from build123d import *

# Parameters (mm, degrees)
F0_R     = 6.35
F1_DEPTH = 12.7
F2_R     = 3.175
F3_DEPTH = 25.4
F4_SIZE  = 3.17499
F5_R     = 3.175
F6_DEPTH = 12.7


# Not quite as in the source:
# - a fillet or chamfer is up to 0.001 mm smaller than in the source, because OpenCascade refuses the exact size


with BuildPart() as f1:
    # F0 (on Top) → F1 (new body, symmetric)
    with BuildSketch(Plane.XY):
        Circle(F0_R)
    extrude(amount=F1_DEPTH, both=True)

    # F2 (on Top) → F3 (join, symmetric)
    with BuildSketch(Plane.XY):
        Circle(F2_R)
    extrude(amount=F3_DEPTH, both=True)

    # F4 (size 3.175 in the source; OpenCascade refuses exactly that, so slightly less here)
    f4_edges = [f1.edges().sort_by_distance(p)[0] for p in [
        (-6.35, 0, -12.7),
        (-6.35, 0, 12.7),
    ]]
    chamfer(f4_edges, length=F4_SIZE)

    # F5 (on Right) → F6 (cut, symmetric)
    with BuildSketch(Plane.YZ):
        Circle(F5_R)
    extrude(amount=F6_DEPTH, both=True, mode=Mode.SUBTRACT)


solid = f1.part
Check sheet for the modelled part. Datum: model origin and axes. Units: mm. A direction names the side the tool comes from. Coordinates: 2 decimals unless noted, no trailing zeros. Loops run counter-clockwise (first coordinate to the right, second up) from the corner with the lowest first, then second, coordinate; pieces in that order, holes last. Notation, with made-up numbers: (-0.75, 19) -> (40.25, 19) arc R34 ccw to (40.25, 57) -> close; hole circle Ø8 at (-18, 17.5). An arc over 180 degrees is marked (long way). Write item = value, one per line. Start each with the question number.
1. Section check C-C on z = 19. Record the cut outline in (x, y) (3 decimals), then the cut area to 3 significant figures.
2. Section check D-D on z = 0. Record the cut outline in (x, y) (3 decimals).
3. Material ranges on line 1 (Z direction, x = -2.75, y = 0) (3 decimals); line 2 (Z direction, x = 1.25, y = 2.5); line 3 (Y direction, x = -1.5, z = 0) (3 decimals), recorded low to high.
4. Depth check by flat-ended pin: P1, Ø5, axis at x = 3, y = -5, coming from the -Z side; P2, Ø3, axis at x = -5, z = 9.5, coming from the +Y side; P3, Ø2, axis at x = 2.5, y = 4.5, coming from the -Z side; P4, Ø5.5, axis at y = 0, z = 0, coming from the +X side. Enter the tip coordinate at first touch or a pass-through.
5. Tool access check on faces 4 (the cylindrical face through (-5.04, -3.86, 0.13)), 5 (the cylindrical face through (-0.69, -3.1, 19.14)), 6 (the cylindrical face through (-0.69, -3.1, -18.96)). Record the directions out of +Z, -Z, +X, -X, +Y, -Y that give a thin tool (end or side, any length) a straight path to the whole face; none if there is none.
6. Draft check along Z on faces 1 (the flat face through (0, 0, -25.4)), 2 (the conical face through (-2.642, -2.026, 12.546)), 3 (the cylindrical face through (0.09, 3.03, 0.95)). Enter one of: released by +Z, released by -Z, zero draft, split by the parting line, or undercut.
Responses:
q1.outline = circle Ø6.35 at (0, 0)
q1.area = 31.7 mm2
q2.outline = (-5.499, -3.175) arc R6.35 ccw to (5.499, -3.175) -> close; (-5.499, 3.175) -> (5.499, 3.175) arc R6.35 ccw to start
q3.line_1 = -25.4 to -3.175, 3.175 to 25.4
q3.line_2 = -25.4 to -1.96, 1.96 to 25.4
q3.line_3 = -6.17 to -3.175, 3.175 to 6.17
q4.P1 = -12.54
q4.P2 = 5.3
q4.P3 = -11.73
q4.P4 = through
q5.face_4 = +Z, -Z
q5.face_5 = +Z
q5.face_6 = -Z
q6.face_1 = released by -Z
q6.face_2 = released by +Z
q6.face_3 = undercut
